Geometry: final body of the model. Coordinates: model frame, mm. A direction names the side the tool comes from. Give positions to 0.01 mm unless a question says otherwise; leave off trailing zeros. Write each loop counter-clockwise with the first axis right and the second up, starting at its lowest first coordinate (ties: lowest second). Pieces come first, ordered by that corner, then holes. Notation, with made-up numbers: M 39,-19 L 60,-19 A22 ccw 60,14 Z; hole C -15.75,77 d6. An arc over 180 degrees is marked long. One line per question, with ' | ' between items.
from build123d import *

# Parameters (mm, degrees)
F0_R     = 10
F1_DEPTH = 25


with BuildPart() as f1:
    # F0 (on Top) → F1 (new body)
    with BuildSketch(Plane.XY):
        with BuildLine():
            ThreePointArc((41.091912, -23.646501), (36.091912, -18.646501), (31.091912, -23.646501))
            ThreePointArc((31.091912, -23.646501), (36.091912, -28.646501), (41.091912, -23.646501))
        make_face()
        with BuildLine():
            ThreePointArc((-8.908088, 1.377323), (-7.85236, 5.849459), (-4.908088, 9.377323))
            ThreePointArc((-4.908088, 9.377323), (-13.908088, 36.377323), (-22.908088, 9.377323))
            ThreePointArc((-22.908088, 9.377323), (-19.963816, 5.849459), (-18.908088, 1.377323))
            Line((-18.908088, 1.377323), (-18.908088, -10.417745))
            ThreePointArc((-18.908088, -10.417745), (-19.553944, -13.953278), (-21.408088, -17.032123))
            ThreePointArc((-21.408088, -17.032123), (-22.858864, -28.105605), (-13.145628, -33.617392))
            Line((-13.145628, -33.617392), (36.086, -33.646499))
            ThreePointArc((36.086, -33.646499), (46.091625, -23.57069), (35.934383, -13.647742))
            Line((35.934383, -13.647742), (1.099337, -13.673606))
            ThreePointArc((1.099337, -13.673606), (-5.97653, -10.747301), (-8.908088, -3.673609))
            Line((-8.908088, -3.673609), (-8.908088, 1.377323))
        make_face()
        with BuildLine():
            ThreePointArc((-8.908088, -23.646501), (-17.443622, -27.182035), (-13.908088, -18.646501))
            ThreePointArc((-13.908088, -18.646501), (-10.372554, -20.110967), (-8.908088, -23.646501))
        make_face(mode=Mode.SUBTRACT)
        with BuildLine():
            ThreePointArc((-13.908088, -13.646501), (-13.474473, -13.655907), (-13.041674, -13.684105))
            Line((-13.041674, -13.684105), (-13.908088, -13.684105))
            Line((-13.908088, -13.684105), (-14.774502, -13.684105))
            ThreePointArc((-14.774502, -13.684105), (-14.341703, -13.655907), (-13.908088, -13.646501))
        make_face(mode=Mode.SUBTRACT)
        with BuildLine():
            ThreePointArc((41.091912, -23.646501), (36.091912, -28.646501), (31.091912, -23.646501))
            ThreePointArc((31.091912, -23.646501), (36.091912, -18.646501), (41.091912, -23.646501))
        make_face(mode=Mode.SUBTRACT)
        with Locations((-13.908088, 21.377323)):
            Circle(F0_R, mode=Mode.SUBTRACT)
    extrude(amount=F1_DEPTH)


solid = f1.part
(1) Material intervals for L1, parallel to Y at x = -6, z = 23; L2, parallel to X at y = 21.5, z = 5.75; L3, parallel to X at y = -27, z = 16.25, sorted ascending. Write a range as [from, to].
Working result:
L1: y = [-33.62, -10.72], [8.43, 15.26], [27.5, 34.12] | L2: x = [-28.91, -23.91], [-3.91, 1.09] | L3: x = [-23.33, -17.62], [-10.2, 32.38], [39.8, 45.51]
(2) Cut plane A-A, the plane x = 40. Return loops of the section in (y, z), then the cut area to 3 significant figures.
Working result:
outline: M -32.85,0 L -26.77,0 L -26.77,25 L -32.85,25 Z; M -20.53,0 L -14.44,0 L -14.44,25 L -20.53,25 Z | area: 304 mm^2
(3) First-contact query: P1, Ø5, axis at y = 27, z = 8, coming from the +X side; P2, Ø2, axis at x = 37.5, z = 5, coming from the -Y side; P3, Ø6, axis at y = -26, z = 12, coming from the -X side. Flat tips, straight axial feed; report the tip coordinate or a pass-through.
Working result:
P1: stops at x = 0.76 | P2: stops at y = -33.64 | P3: stops at x = -23.91
(4) Set-up query: faces 4 (the face through (31.323, -22.145, 12.325)), 5 (the face through (-18.908, -4, 12)), 6 (the face through (-7.88, 5.79, 12.32)). Return all of +Z, -Z, +X, -X, +Y, -Y with unobstructed straight access to the full face (end or side cutting, diameter ignored); none if empty.
Working result:
face 4: +Z, -Z | face 5: +Z, -Z, -X | face 6: +Z, -Z, +X
(5) Cut plane D-D, the plane z = 20. Return loops of the section in (x, y).
Working result:
outline: M -22.91,9.38 A10 cw -18.91,1.38 L -18.91,-10.42 A10 cw -21.41,-17.03 A10 ccw -13.15,-33.62 L 36.09,-33.65 A10 ccw long 35.93,-13.65 L 1.1,-13.67 A10 cw -8.91,-3.67 L -8.91,1.38 A10 cw -4.91,9.38 A15 ccw long Z; hole C -13.91,21.38 d20; hole C -13.91,-23.65 d10; hole M -14.77,-13.68 L -13.04,-13.68 A10 ccw -13.91,-13.65 A10 ccw Z; hole C 36.09,-23.65 d10
(6) Cut plane C-C, the plane y = 13. Return loops of the section in (x, z).
Working result:
outline: M -26.35,0 L -19.37,0 L -19.37,25 L -26.35,25 Z; M -8.45,0 L -1.47,0 L -1.47,25 L -8.45,25 Z
(7) Draft query along Y for faces 1 (the face through (-5.898, -10.825, 12.325)), 2 (the face through (0, -14, 0)), 3 (the face through (46.09, -23.79, 12.32)). Return one class per face: released by +Y, released by -Y, zero draft, split by the parting line, or undercut.
Working result:
face 1: undercut | face 2: zero draft | face 3: split by the parting line
(8) Cut plane B-B, the plane y = -21. Return loops of the section in (x, z).
Working result:
outline: M -23.55,0 L -18.15,0 L -18.15,25 L -23.55,25 Z; M -9.67,0 L 31.85,0 L 31.85,25 L -9.67,25 Z; M 40.33,0 L 45.74,0 L 45.74,25 L 40.33,25 Z
